Work out the finished part from the listing and answer in its coordinate system (mm). A direction names the side the tool comes from. Coordinates: 2 decimals unless noted, no trailing zeros. Loops run counter-clockwise (first coordinate to the right, second up) from the corner with the lowest first, then second, coordinate; pieces in that order, holes last. Notation, with made-up numbers: (-25, 29) -> (32, 29) arc R21 ccw to (32, 49) -> close; hole circle Ø6 at (-31.5, 35). An arc over 180 degrees is marked (long way). Answer as CSV lines item,"result".
```python
from build123d import *

# Parameters (mm, degrees)
Y_KSEKLIK_EKSTR_ZYON1_DEPTH = 5
Y_KSEKLIK_EKSTR_ZYON2_DEPTH = 5
IZIM3_R                     = 1.25
KES_EKSTR_ZYON1_DEPTH       = 5
IZIM4_R                     = 1.25
KES_EKSTR_ZYON2_DEPTH       = 5


with BuildPart() as part:
    # Çizim1 → Yükseklik-Ekstrüzyon1 (new body)
    with BuildSketch(Plane.XY):
        with BuildLine():
            Line((0, 0), (20, 0))
            ThreePointArc((20, 0), (10, 10), (0, 0))
        make_face()
    extrude(amount=Y_KSEKLIK_EKSTR_ZYON1_DEPTH)

    # Çizim2 → Yükseklik-Ekstrüzyon2 (add)
    with BuildSketch(Plane.XZ):
        with BuildLine():
            Line((0, 15), (0, 0))
            Line((0, 0), (20, 0))
            Line((20, 0), (20, 15))
            ThreePointArc((20, 15), (10, 25), (0, 15))
        make_face()
    extrude(amount=Y_KSEKLIK_EKSTR_ZYON2_DEPTH)

    # Çizim3 → Kes-Ekstrüzyon1 (cut)
    with BuildSketch(Plane.XY.offset(5)):
        with Locations((10, 5)):
            Circle(IZIM3_R)
    extrude(amount=-KES_EKSTR_ZYON1_DEPTH, mode=Mode.SUBTRACT)

    # Çizim4 → Kes-Ekstrüzyon2 (cut)
    with BuildSketch(Plane(origin=(0, 0, 0), x_dir=(1, 0, 0), z_dir=(0, 1, 0))):
        with Locations(Location((10, -15, 0), (0, 0, 270))):
            Circle(IZIM4_R)
    extrude(amount=-KES_EKSTR_ZYON2_DEPTH, mode=Mode.SUBTRACT)


solid = part.part
```
(1) A cutting plane is placed at D-D, the plane x = 2. Write down the section's boundary in (y, z).
Computed values:
outline,"(-5, 0) -> (6, 0) -> (6, 5) -> (0, 5) -> (0, 21) -> (-5, 21) -> close"
(2) Which of the six approach directions +Z, -Z, +X, -X, +Y, -Y give full straight-line access (tool end or side, diameter ignored) to faces 5 (the face through (11.24, -2.46, 14.84)), 6 (the face through (10, 3, 5))?
Computed values:
face 5,"+Y, -Y"
face 6,"+Z, +X, -X, +Y"
(3) A cutting plane is placed at B-B, the plane y = -3.5. Write down the section's boundary in (x, z).
Computed values:
outline,"(0, 0) -> (20, 0) -> (20, 15) arc R10 ccw to (0, 15) -> close; hole circle Ø2.5 at (10, 15)"
(4) For a pull along Y with two mould halves and no side action, classify faces 1 (the face through (10, 0, 13)), 2 (the face through (9.01, 4.24, 2.54)), 3 (the face through (20, -2, 7)), 4 (the face through (10, -5, 13)) as pulls with the +Y half, pulls with the -Y half, needs draft (parallel to the pull), parting line crosses it, or undercut.
Computed values:
face 1,"pulls with the +Y half"
face 2,"undercut"
face 3,"needs draft"
face 4,"pulls with the -Y half"
(5) A cutting plane is placed at C-C, the plane y = 5. Write down the section's boundary in (x, z), and give its area (3 significant figures).
Computed values:
outline,"(1.34, 0) -> (8.75, 0) -> (8.75, 5) -> (1.34, 5) -> close; (11.25, 0) -> (18.66, 0) -> (18.66, 5) -> (11.25, 5) -> close"
area,"74.1 mm2"
(6) Consider line 1 along Y through (x, z) = (10, 3.25); line 2 along Y through (x, z) = (15.75, 7); line 3 along Z through (x, y) = (12, 5). Determine where each line is inside the solid, lowest interval first.
Computed values:
line 1,"-5 to 3.75, 6.25 to 10"
line 2,"-5 to 0"
line 3,"0 to 5"
(7) Flat-ended cylindrical pins translate along their axes: pin 1 Ø10 at (x, z) = (10.5, 12.5) entering from +Y; pin 2 Ø3 at (x, y) = (10, 5) entering from +Z; pin 3 Ø4 at (y, z) = (2.5, 5.5) entering from +X. Find the tip coordinate at first contact, or state that the pin passes through.
Computed values:
pin 1,"y = 0"
pin 2,"z = 5"
pin 3,"x = 19.98"
(8) A cutting plane is placed at A-A, the plane x = 10. Write down the section's boundary in (y, z), and give its area (3 significant figures).
Computed values:
outline,"(-5, 0) -> (3.75, 0) -> (3.75, 5) -> (0, 5) -> (0, 13.75) -> (-5, 13.75) -> close; (-5, 16.25) -> (0, 16.25) -> (0, 25) -> (-5, 25) -> close; (6.25, 0) -> (10, 0) -> (10, 5) -> (6.25, 5) -> close"
area,"150 mm2"
